Input: dimensioned drawing with shaded views. Units: mm. Origin: part minimum x, y, z. Round coordinates to 2 decimals unless told otherwise and drop trailing zeros. Write each loop counter-clockwise with the first axis right and the second up, starting at its lowest first coordinate (ties: lowest second). Pieces come first, ordered by that corner, then holes. Notation, with made-up numbers: M -10,84.5 L 6,84.5 A33 cw 6,113.5 Z; hole C 51.5,7.25 d10. An arc over 180 degrees is marked long. Answer in a Markdown table with one row per item. Add a question column.
Item 1: Cut plane B-B on z = 32.5. Return loops of the section in (x, y), and give its area (3 significant figures).
Item 2: Material intervals for probe 1 along Y at (x, z) = (76.5, 75); probe 2 along X at (y, z) = (62.5, 48), sorted ascending.
Item 3: Cut plane C-C on z = 92. Return loops of the section in (x, y), and give its area (3 significant figures).
Item 4: Cut plane A-A on x = 22. Return loops of the section in (y, z).
Item 5: Contact query for a flat-ended pin moving along its axis: pin 1 (10 mm diameter, centred on x = 43.5, y = 59, fed in from -Z). Output: stop coordinate, or through.
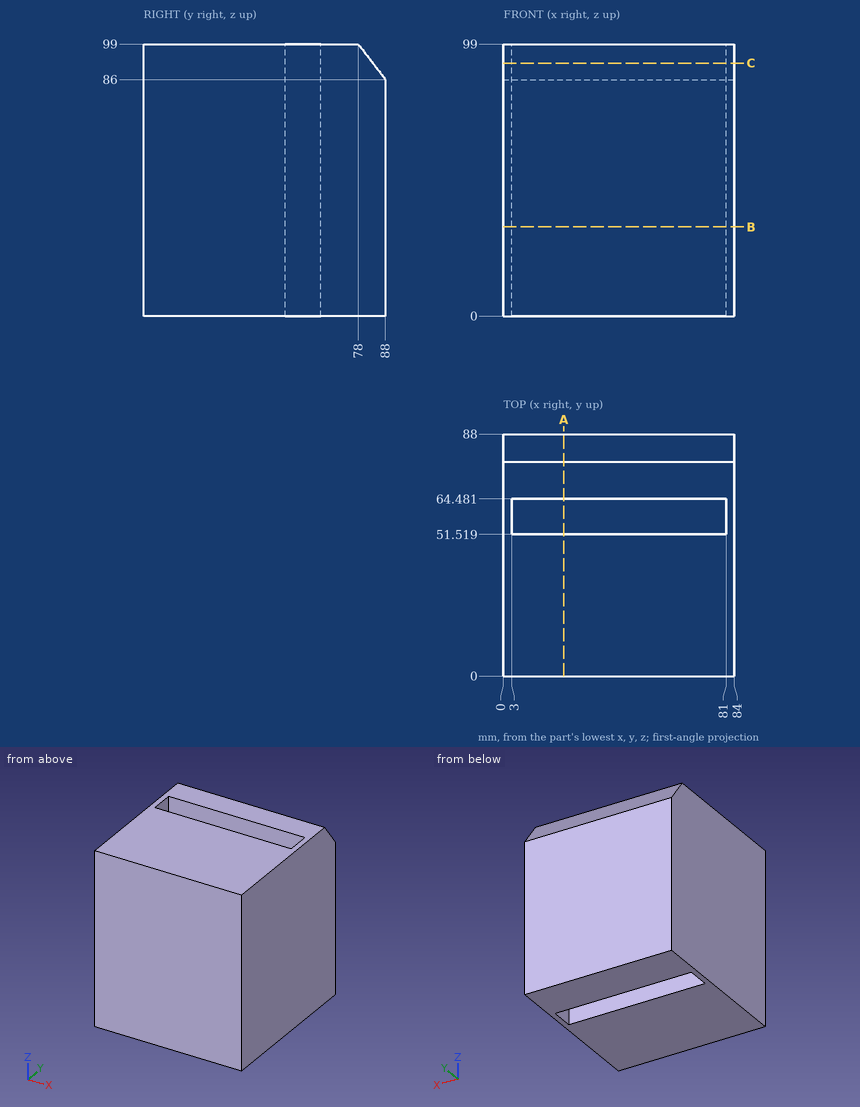
Results below:
| question | item | result |
|---|---|---|
| 1 | outline | M 0,0 L 84,0 L 84,88 L 0,88 Z; hole M 3,51.52 L 81,51.52 L 81,64.48 L 3,64.48 Z |
| 1 | area | 6,380 mm2 |
| 2 | probe 1 | 0 to 51.52, 64.48 to 88 |
| 2 | probe 2 | 0 to 3, 81 to 84 |
| 3 | outline | M 0,0 L 84,0 L 84,83.38 L 0,83.38 Z; hole M 3,51.52 L 81,51.52 L 81,64.48 L 3,64.48 Z |
| 3 | area | 5,990 mm2 |
| 4 | outline | M 0,0 L 51.52,0 L 51.52,99 L 0,99 Z; M 64.48,0 L 88,0 L 88,86 L 78,99 L 64.48,99 Z |
| 5 | pin 1 | through |
